from build123d import *

# Parameters (mm, degrees)
SKETCH1_R           = 12.7
SKETCH1_R_2         = 2.6035
BOSS_EXTRUDE1_DEPTH = 6.35


with BuildPart() as part:
    # Sketch1 → Boss-Extrude1 (new body)
    with BuildSketch(Plane.ZY.offset(-33.3375)):
        with BuildLine():
            ThreePointArc((26.955926991, 186.931527045), (24.401493508, 181.09830314), (18.382320409, 179.019556705))
            ThreePointArc((18.382320409, 179.019556705), (8.384293755, 175.340660282), (4.705397332, 165.342633628))
            ThreePointArc((4.705397332, 165.342633628), (2.626650896, 159.323460528), (-3.206573009, 156.769027045))
            ThreePointArc((-3.206573009, 156.769027045), (-9.039796914, 159.323460528), (-11.118543349, 165.342633628))
            ThreePointArc((-11.118543349, 165.342633628), (-14.797439772, 175.340660282), (-24.795466426, 179.019556705))
            ThreePointArc((-24.795466426, 179.019556705), (-30.814639526, 181.09830314), (-33.369073009, 186.931527045))
            ThreePointArc((-33.369073009, 186.931527045), (-30.814639526, 192.76475095), (-24.795466426, 194.843497386))
            ThreePointArc((-24.795466426, 194.843497386), (-14.797439772, 198.522393809), (-11.118543349, 208.520420462))
            ThreePointArc((-11.118543349, 208.520420462), (-9.039796914, 214.539593562), (-3.206573009, 217.094027045))
            ThreePointArc((-3.206573009, 217.094027045), (2.626650896, 214.539593562), (4.705397332, 208.520420462))
            ThreePointArc((4.705397332, 208.520420462), (8.384293755, 198.522393809), (18.382320409, 194.843497386))
            ThreePointArc((18.382320409, 194.843497386), (24.401493508, 192.76475095), (26.955926991, 186.931527045))
        make_face()
        with Locations((-3.206573009, 186.931527045)):
            Circle(SKETCH1_R, mode=Mode.SUBTRACT)
        with Locations((19.018426991, 186.931527045)):
            Circle(SKETCH1_R_2, mode=Mode.SUBTRACT)
        with Locations((-3.206573009, 164.706527045)):
            Circle(SKETCH1_R_2, mode=Mode.SUBTRACT)
        with Locations((-25.431573009, 186.931527045)):
            Circle(SKETCH1_R_2, mode=Mode.SUBTRACT)
        with Locations((-3.206573009, 209.156527045)):
            Circle(SKETCH1_R_2, mode=Mode.SUBTRACT)
    extrude(amount=BOSS_EXTRUDE1_DEPTH)


solid = part.part
Here's how the part is built. I have some questions about the finished solid (model axes, mm). Round coordinates to 2 decimals unless told otherwise and drop trailing zeros. Loops run counter-clockwise (first coordinate to the right, second up) from the corner with the lowest first, then second, coordinate; pieces in that order, holes last.
1. If I drill on line 1 along Y through (x, z) = (28.25, 19); line 2 along Y through (x, z) = (31, -9); line 3 along Z through (x, y) = (31.75, 166), over which ranges is the centre line in solid material (lowest first)?
Answer list:
line 1: y = 178.99 to 184.33, 189.53 to 194.87
line 2: y = 159.28 to 175.63, 198.23 to 214.58
line 3: z = -11.08 to -5.47, -0.95 to 4.67
2. If we section it at B-B on z = 1.5: Write out the boundary of the cut face in (x, y), plus the area to 3 significant figures.
Answer list:
outline: (26.99, 158.31) - (33.34, 158.31) - (33.34, 175.14) - (26.99, 175.14) - close; (26.99, 198.73) - (33.34, 198.73) - (33.34, 215.55) - (26.99, 215.55) - close
area: 214 mm2
3. If we section it at A-A on y = 175: Write out the boundary of the cut face in (x, z), plus the area to 3 significant figures.
Answer list:
outline: (26.99, -14.47) - (33.34, -14.47) - (33.34, -7.56) - (26.99, -7.56) - close; (26.99, 1.14) - (33.34, 1.14) - (33.34, 8.06) - (26.99, 8.06) - close
area: 87.8 mm2
4. If we section it at D-D on z = 11: Write out the boundary of the cut face in (x, y), plus the area to 3 significant figures.
Answer list:
outline: (26.99, 177.35) - (33.34, 177.35) - (33.34, 196.51) - (26.99, 196.51) - close
area: 122 mm2
5. For P1, Ø3, axis at x = 32.5, z = 19.5, coming from the -Y side; P2, Ø1.5, axis at x = 30, y = 208.5, coming from the -Z side; P3, Ø1, axis at x = 32, y = 205, coming from the +Z side, each with a flat end and sliding along its axis, tell me the tip position at first contact or that it passes through.
Answer list:
P1: stops at y = 178.99
P2: stops at z = -11.14
P3: stops at z = 5.02
6. We'd pull the mould along Z, two halves only. Please class faces 1 (the face through (33.338, 176, -10)), 2 (the face through (30.207, 199.523, -4.86)): +Z half, -Z half, draft (parallel to the pull), parting line (faces both ways), or undercut.
Answer list:
face 1: draft
face 2: undercut
